Geometry check sheet. Reference: the model listing, model coordinates, mm. Round coordinates to 2 decimals unless told otherwise and drop trailing zeros. Loops run counter-clockwise (first coordinate to the right, second up) from the corner with the lowest first, then second, coordinate; pieces in that order, holes last. Notation, with made-up numbers: (-20.75, -16.5) - (36.25, -16.5) arc R30 cw to (36.25, 7.5) - close; hole circle Ø11 at (-15, 85.25). An arc over 180 degrees is marked (long way). Answer in a Markdown table with one row per item. Add a question column.
Autodesk Fusion 360 part; units mm, degrees
sketch "Sketch1" plane through (0, 0, 0) normal (0, 0, 1) x (1, 0, 0)
  line L0 (11.2333, -2) -> (15, -2)
  line L1 (15, -2) -> (15, -102)
  line L2 (15, -102) -> (0, -102)
  line L3 (0, -102) -> (0, -10.3)
  line L4 (3.55, -6.2) -> (3.55, -10.3)
  line L5 (3.55, -10.3) -> (0, -10.3)
  line L6 (3.55, -6.2) -> (3.55, -6.0626)
  spline S0 degree 5 poles (0.0005, -6.2) (0.0004, -6.2) (0.0003, -6.2) (0.0002, -6.2) (0.0001, -6.2) (0, -6.2) knots 0.999983 0.999983 0.999983 0.999983 0.999983 0.999983 1 1 1 1 1 1
  spline S1 degree 5 poles (11.2333, -2) (11.2207, -2.1206) (11.1821, -2.3832) (11.0805, -2.7956) (10.8375, -3.3499) (10.3193, -3.992) (9.5498, -4.5477) (8.6121, -5.0047) (7.56, -5.3794) (6.3963, -5.6787) (5.3546, -5.8645) (4.4953, -5.9743) (3.8803, -6.0347) (3.558, -6.0619) (3.55, -6.0626) knots 0.274949 0.274949 0.274949 0.274949 0.274949 0.274949 0.333333 0.4 0.466667 0.533333 0.6 0.666667 0.733333 0.8 0.866667 0.86836 0.86836 0.86836 0.86836 0.86836 0.86836
  dimension "d4" = 3.55
  dimension "d5" = 4.1
revolve "Revolve1" add sketch "Sketch1" angle 360 about axis through (0, 1.75, 0) along (0, 1, 0)
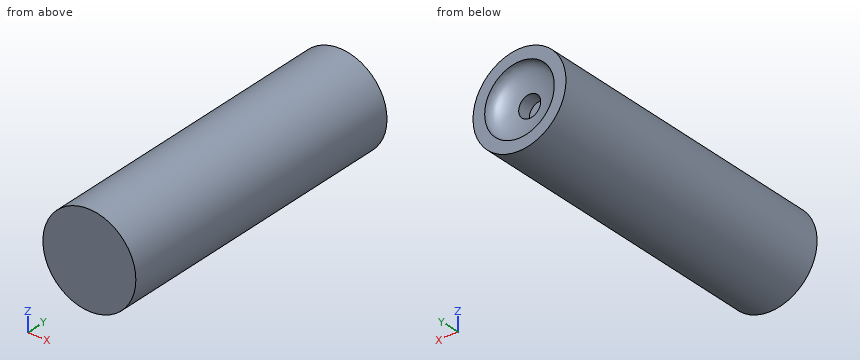
Q1. Scan lines: line 1 (X direction, y = -8.75, z = 0); line 2 (X direction, y = -34, z = -13). Record each from-to range of solid material in increasing order. Write a range as from..to.
Q2. Depth check by flat-ended pin: P1, Ø10, axis at x = 9, z = 5.5, coming from the +Y side; P2, Ø5.5, axis at x = 0, z = 0, coming from the +Y side; P3, Ø10, axis at x = 6.5, y = -38.5, coming from the -Z side; P4, Ø5, axis at y = -43.5, z = -8.5, coming from the +X side. Enter the tip coordinate at first touch or a pass-through.
Q3. Cross-section at B-B, the plane x = 13.25. Enter the section's corners in (y, z).
Q4. Cross-section at A-A, the plane y = -45.5. Enter the section's corners in (x, z), plus the area to 3 significant figures.
Check sheet entries:
| question | item | result |
|---|---|---|
| 1 | line 1 | -15..-3.55, 3.55..15 |
| 1 | line 2 | -7.48..7.48 |
| 2 | P1 | y = -2 |
| 2 | P2 | y = -10.3 |
| 2 | P3 | z = -14.92 |
| 2 | P4 | x = 13.75 |
| 3 | outline | (-102, -7.03) - (-2, -7.03) - (-2, 7.03) - (-102, 7.03) - close |
| 4 | outline | circle Ø30 at (0, 0) |
| 4 | area | 707 mm² |
